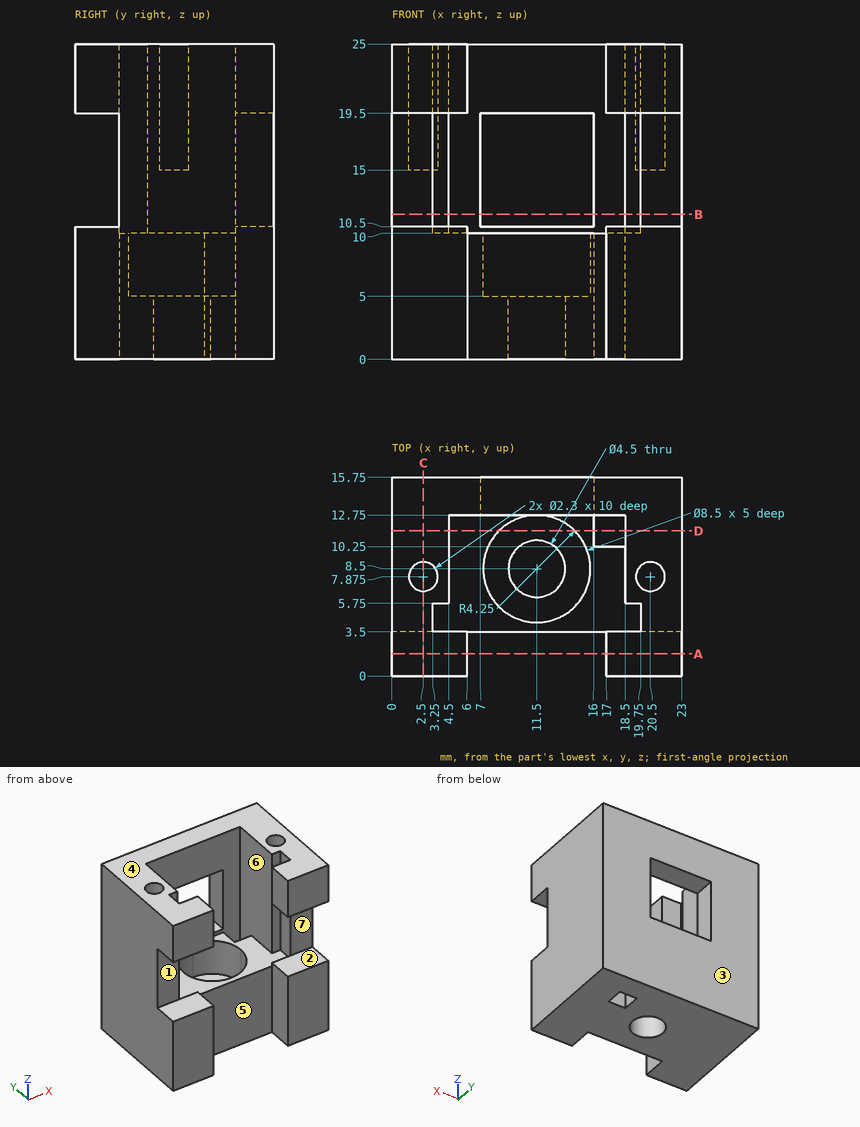
Geometry: see drawing. Coordinates: mm, zero at the bounding-box minimum. A direction names the side the tool comes from. Give positions to 0.01 mm unless a question says otherwise; leave off trailing zeros. Write each loop counter-clockwise with the first axis right and the second up, starting at its lowest first coordinate (ties: lowest second). Pieces come first, ordered by that corner, then holes. Notation, with made-up numbers: M 7.5,43 L 20.5,43 A7 cw 20.5,54 Z; hole C 6.5,16 d7. An arc over 180 degrees is marked long. Answer in a Markdown table with one row per item. Add a question column.
(1) Ray query, line 1 (Y direction, x = 2.5, z = 22.25) (3 decimals); line 2 (Y direction, x = 11.5, z = 8.1); line 3 (X direction, y = 1.25, z = 6). Return the intervals inside material, ascending.
(2) Section B-B on z = 11.5. Return loops of the section in (x, y).
(3) Section A-A on y = 1.75. Return loops of the section in (x, z), and give its area (3 significant figures).
(4) First-contact query: pin 1 (4 mm diameter, centred on x = 11, z = 8, fed in from -Y); pin 2 (1.4 mm diameter, centred on x = 20.5, y = 7.875, fed in from +Z). Flat tips, straight axial feed; report the tip coordinate or a pass-through.
(5) Section D-D on y = 11.5. Return loops of the section in (x, z).
(6) Section C-C on x = 2.5. Return loops of the section in (y, z) (3 decimals), and give its area (3 significant figures).
(7) Mould query, pull axis Z, two halves, no side actions, for the marked faces 1, 2, 3 and 4. Classes: +Z half, -Z half, draft (parallel to the pull), parting line (faces both ways), or undercut.
(8) Reachability of the marked faces 5, 6 and 7 from +Z, -Z, +X, -X, +Y, -Y: full face, straight path, thin tool, end or side. Return the list, or none.
Result set:
| question | item | result |
|---|---|---|
| 1 | line 1 | y = 0 to 6.725, 9.025 to 15.75 |
| 1 | line 2 | y = 3.5 to 4.25, 12.75 to 15.75 |
| 1 | line 3 | x = 0 to 6, 17 to 23 |
| 2 | outline | M 0,3.5 L 3.25,3.5 L 3.25,5.75 L 4.5,5.75 L 4.5,12.75 L 7,12.75 L 7,15.75 L 0,15.75 Z; M 16,12.75 L 18.5,12.75 L 18.5,5.75 L 19.75,5.75 L 19.75,3.5 L 23,3.5 L 23,15.75 L 16,15.75 Z |
| 3 | outline | M 0,0 L 6,0 L 6,10.5 L 0,10.5 Z; M 0,19.5 L 6,19.5 L 6,25 L 0,25 Z; M 17,0 L 23,0 L 23,10.5 L 17,10.5 Z; M 17,19.5 L 23,19.5 L 23,25 L 17,25 Z |
| 3 | area | 192 mm^2 |
| 4 | pin 1 | stops at y = 3.5 |
| 4 | pin 2 | stops at z = 15 |
| 5 | outline | M 0,0 L 16,0 L 16,10 L 14.51,10 L 14.51,5 L 8.49,5 L 8.49,10 L 4.5,10 L 4.5,25 L 0,25 Z; M 18.5,0 L 23,0 L 23,25 L 18.5,25 Z |
| 6 | outline | M 0,0 L 15.75,0 L 15.75,25 L 9.025,25 L 9.025,15 L 6.725,15 L 6.725,25 L 0,25 L 0,19.5 L 3.5,19.5 L 3.5,10.5 L 0,10.5 Z |
| 6 | area | 339 mm^2 |
| 7 | face 1 | undercut |
| 7 | face 2 | undercut |
| 7 | face 3 | draft |
| 7 | face 4 | +Z half |
| 8 | face 5 | +Z, -Z, -Y |
| 8 | face 6 | +Z |
| 8 | face 7 | +X, -X, -Y |
